Check sheet for the modelled part. Datum: model origin and axes. Units: mm. Give positions to 0.01 mm unless a question says otherwise; leave off trailing zeros. Order: outer loops, then holes, each group sorted by start corner. A loop starts at its lowest first (then second) coordinate and runs counter-clockwise, first axis right, second up. Notation, with made-up numbers: (-25, 69) -> (7, 69) arc R21 ccw to (7, 89) -> close; hole circle Ø7 at (4.25, 40). An arc over 180 degrees is marked (long way). Answer in a Markdown table with one row per item. Add a question column.
(1) Cross-section at C-C (z = 0.55). State how many separate pieces and enclosed holes the cut face has, then the cut area to 3 significant figures.
(2) Cross-section at B-B (x = 0). Record the cut outline in (y, z) (3 decimals).
(3) Go/stop test with flat-tipped pins: pin 1 (10 mm diameter, centred on x = 49.5, y = -43, fed in from -Z); pin 2 (3 mm diameter, centred on x = -63.24, y = 36.51, fed in from +Z); pin 3 (1 mm diameter, centred on y = 67, z = 2, fed in from -X); pin 4 (1 mm diameter, centred on y = -64.5, z = 1, fed in from -X). Record where each tip stops, or that it passes through.
(4) Cross-section at A-A (y = 0). Record the cut outline in (x, z) (3 decimals).
(5) Thickness scan on L1, parallel to Y at x = 0, z = 0.75 (3 decimals); L2, parallel to Y at x = 15, z = 1.2; L3, parallel to X at y = -40, z = 0.75. Record the ranges inside material, lowest first. Write a range as [from, to].
```python
from build123d import *

# Parameters (mm, degrees)
F0_R            = 76.2
F0_R_2          = 1.8288
F0_R_3          = 53.975
F1_DEPTH        = 3.175
F3_DEPTH        = 3.175
F3_COPIES_COUNT = 6


# Not quite as in the source:
# - a pattern or mirror of a feature is missing from the dataset's text; its kind, count and spacing are read off the source's solid


with BuildPart() as f1:
    # F0 (on Top) → F1 (new body)
    with BuildSketch(Plane.XY):
        Circle(F0_R)
        with Locations((-49.4933518263, -28.575)):
            Circle(F0_R_2, mode=Mode.SUBTRACT)
        with Locations((0, -73.025)):
            Circle(F0_R_2, mode=Mode.SUBTRACT)
        with Locations((49.4933518263, -28.575)):
            Circle(F0_R_2, mode=Mode.SUBTRACT)
        with Locations((-63.2415051114, 36.5125)):
            Circle(F0_R_2, mode=Mode.SUBTRACT)
        Circle(F0_R_3, mode=Mode.SUBTRACT)
        with Locations((63.2415051114, 36.5125)):
            Circle(F0_R_2, mode=Mode.SUBTRACT)
        with Locations((0, 57.15)):
            Circle(F0_R_2, mode=Mode.SUBTRACT)
    extrude(amount=F1_DEPTH)

    # F2 (on face) → F3 (cut, through all)
    with BuildSketch(Plane.XY.offset(3.175)):
        with BuildLine():
            Line((-3.175, 60.2413894262), (-3.175, 69.7778035983))
            ThreePointArc((-3.175, 69.7778035983), (-34.925, 60.4918744543), (-58.8418505364, 37.6385324562))
            Line((-58.8418505364, 37.6385324562), (-50.5830736024, 32.8703253701))
            ThreePointArc((-50.5830736024, 32.8703253701), (-30.1625, 52.2429824833), (-3.175, 60.2413894262))
        make_face()
    f3 = extrude(amount=-F3_DEPTH, mode=Mode.SUBTRACT)

    # F3_copies: F3 ×6 about axis
    f3_copies_axis = Axis((0, 0, 0), (0, 0, 1))
    for i in range(1, F3_COPIES_COUNT):
        add(f3.rotate(f3_copies_axis, i * 360 / F3_COPIES_COUNT), mode=Mode.SUBTRACT)


solid = f1.part
```
Answer below:
| question | item | result |
|---|---|---|
| 1 | separate pieces | 1 |
| 1 | enclosed holes | 13 |
| 1 | area | 5,490 mm² |
| 2 | outline | (-76.2, 0) -> (-74.854, 0) -> (-74.854, 3.175) -> (-76.2, 3.175) -> close; (-71.196, 0) -> (-53.975, 0) -> (-53.975, 3.175) -> (-71.196, 3.175) -> close; (53.975, 0) -> (55.321, 0) -> (55.321, 3.175) -> (53.975, 3.175) -> close; (58.979, 0) -> (76.2, 0) -> (76.2, 3.175) -> (58.979, 3.175) -> close |
| 3 | pin 1 | stops at z = 0 |
| 3 | pin 2 | passes through |
| 3 | pin 3 | stops at x = -37.2 |
| 3 | pin 4 | stops at x = -41.36 |
| 4 | outline | (-76.2, 0) -> (-69.85, 0) -> (-69.85, 3.175) -> (-76.2, 3.175) -> close; (-60.325, 0) -> (-53.975, 0) -> (-53.975, 3.175) -> (-60.325, 3.175) -> close; (53.975, 0) -> (60.325, 0) -> (60.325, 3.175) -> (53.975, 3.175) -> close; (69.85, 0) -> (76.2, 0) -> (76.2, 3.175) -> (69.85, 3.175) -> close |
| 5 | L1 | y = [-76.2, -74.854], [-71.196, -53.975], [53.975, 55.321], [58.979, 76.2] |
| 5 | L2 | y = [-74.71, -68.22], [-58.43, -51.85], [51.85, 58.43], [68.22, 74.71] |
| 5 | L3 | x = [-64.86, -57.26], [-45.16, -36.24], [36.24, 45.16], [57.26, 64.86] |
